Verification items for the finished model (mm, model axes). Coordinates: 2 decimals unless noted, no trailing zeros. Write each loop counter-clockwise with the first axis right and the second up, starting at its lowest first coordinate (ties: lowest second). Pieces come first, ordered by that corner, then holes. Notation, with made-up numbers: M 60.25,8 L 112.25,8 A31 ccw 112.25,44 Z; hole C 61.25,-27 d6. An arc over 180 degrees is marked long. Answer in a Markdown table with one row per item.
Autodesk Inventor part; units mm, degrees
ref_plane "YZ Plane" through (0, 0, 0) normal (1, 0, 0) x (0, 1, 0)
ref_plane "XZ Plane" through (0, 0, 0) normal (0, 1, 0) x (-1, 0, 0)
ref_plane "XY Plane" through (0, 0, 0) normal (0, 0, 1) x (1, 0, 0)
sketch "Sketch1" plane through (0, 0, 0) normal (0, 1, 0) x (-1, 0, 0)
  line L0 (-0.4496, -20) -> (-0.4496, 0)
  line L1 (-41.2289, 0) -> (-41.2289, -20)
  circle A0 centre (13.17, -3) radius 1.05
  circle A1 centre (5.87, -10) radius 1.05
  circle A2 centre (13.17, -17) radius 1.05
  circle A3 centre (26.39, -18) radius 1.05
  circle A4 centre (26.39, -2) radius 1.05
  circle A5 centre (-62.4686, -2.475) radius 1.05
  circle A6 centre (-62.4686, -17.525) radius 1.05
  circle A7 centre (-47.3686, -17.525) radius 1.05
  circle A8 centre (-47.3686, -2.475) radius 1.05
  circle A9 centre (-13.8393, -17) radius 1.5
  circle A10 centre (-13.8393, -3) radius 1.5
  circle A11 centre (-27.8393, -3) radius 1.5
  circle A12 centre (-27.8393, -17) radius 1.5
  arc A13 (32.29, -20) -> (33.29, -19) centre (32.29, -19) ccw
  line L2 (33.29, -19) -> (33.29, -16.4)
  arc A14 (33.29, -1) -> (32.29, 0) centre (32.29, -1) ccw
  line L3 (33.29, -3.6) -> (33.29, -1)
  arc A15 (-73.9686, 0) -> (-74.9686, -1) centre (-73.9686, -1) ccw
  arc A16 (-74.9686, -19) -> (-73.9686, -20) centre (-73.9686, -19) ccw
  line L4 (-74.9686, -1) -> (-74.9686, -3.6)
  line L5 (-74.9686, -16.4) -> (-74.9686, -19)
  arc A17 (33.29, -3.6) -> (33.29, -16.4) centre (33.29, -10) ccw
  arc A18 (-74.9686, -16.4) -> (-74.9686, -3.6) centre (-74.9686, -10) ccw
  line L6 (32.29, -20) -> (-73.9686, -20)
  line L7 (-73.9686, 0) -> (32.29, 0)
  line L8 (-41.6786, -20) -> (-41.6786, 0)
  line L9 (-40.7793, 0) -> (-40.7793, -20)
  line L10 (-0.8993, -20) -> (-0.8993, 0)
  line L11 (0, 0) -> (0, -20)
extrude "Extrusion1" add sketch "Sketch1" against normal blind 1.5
properties part number "CAM_axis_5_top_frame"
1) Sectioned sample at B-B (y = -0.3). Give the number of separate pieces and of enclosed holes in the cut face, then the cut area to 3 significant figures.
Response values:
| item | result |
|---|---|
| separate pieces | 1 |
| enclosed holes | 13 |
| area | 1,980 mm² |
2) Thickness scan on L1, parallel to Z at x = -13.17, y = -0.7; L2, parallel to Z at x = -26.39, y = -1.2; L3, parallel to Z at x = -6, y = -0.4. Record the ranges inside material, lowest first. Write a range as [from, to].
Response values:
| item | result |
|---|---|
| L1 | z = [-20, -18.05], [-15.95, -4.05], [-1.95, 0] |
| L2 | z = [-20, -19.05], [-16.95, -3.05], [-0.95, 0] |
| L3 | z = [-20, -11.04], [-8.96, 0] |
3) Depth check by flat-ended pin: pin 1 (2 mm diameter, centred on x = 58, z = -5, fed in from +Y). Enter the tip coordinate at first touch or a pass-through.
Response values:
| item | result |
|---|---|
| pin 1 | stops at y = 0 |
4) Sectioned sample at C-C (z = -5.5). Record the cut outline in (x, y), then the cut area to 3 significant figures.
Response values:
| item | result |
|---|---|
| outline | M -28.74,-1.5 L 70.42,-1.5 L 70.42,0 L -28.74,0 Z |
| area | 149 mm² |
5) Sectioned sample at A-A (z = -10). Record the cut outline in (x, y), then the cut area to 3 significant figures.
Response values:
| item | result |
|---|---|
| outline | M -26.89,-1.5 L -6.92,-1.5 L -6.92,0 L -26.89,0 Z; M -4.82,-1.5 L 68.57,-1.5 L 68.57,0 L -4.82,0 Z |
| area | 140 mm² |
6) Release check for a two-part mould opening along Z. For faces 1 (the face through (22, -1.5, -10)), 2 (the face through (14.945, -0.74, -15.986)) record: +Z half, -Z half, draft (parallel to the pull), parting line (faces both ways), or undercut.
Response values:
| item | result |
|---|---|
| face 1 | draft |
| face 2 | undercut |
